Check sheet for the drawn part. Datum: minimum x, y, z corner. Units: mm. A direction names the side the tool comes from. Round coordinates to 2 decimals unless told otherwise and drop trailing zeros. Order: outer loops, then holes, each group sorted by start corner. A loop starts at its lowest first (then second) coordinate and runs counter-clockwise, first axis right, second up. Notation, with made-up numbers: (48, 45) -> (99, 45) arc R13 ccw to (99, 66) -> close; hole circle Ø6 at (62.25, -8.5). An arc over 180 degrees is marked (long way). Answer as a JSON object with one key per item and string values. Group by question number.
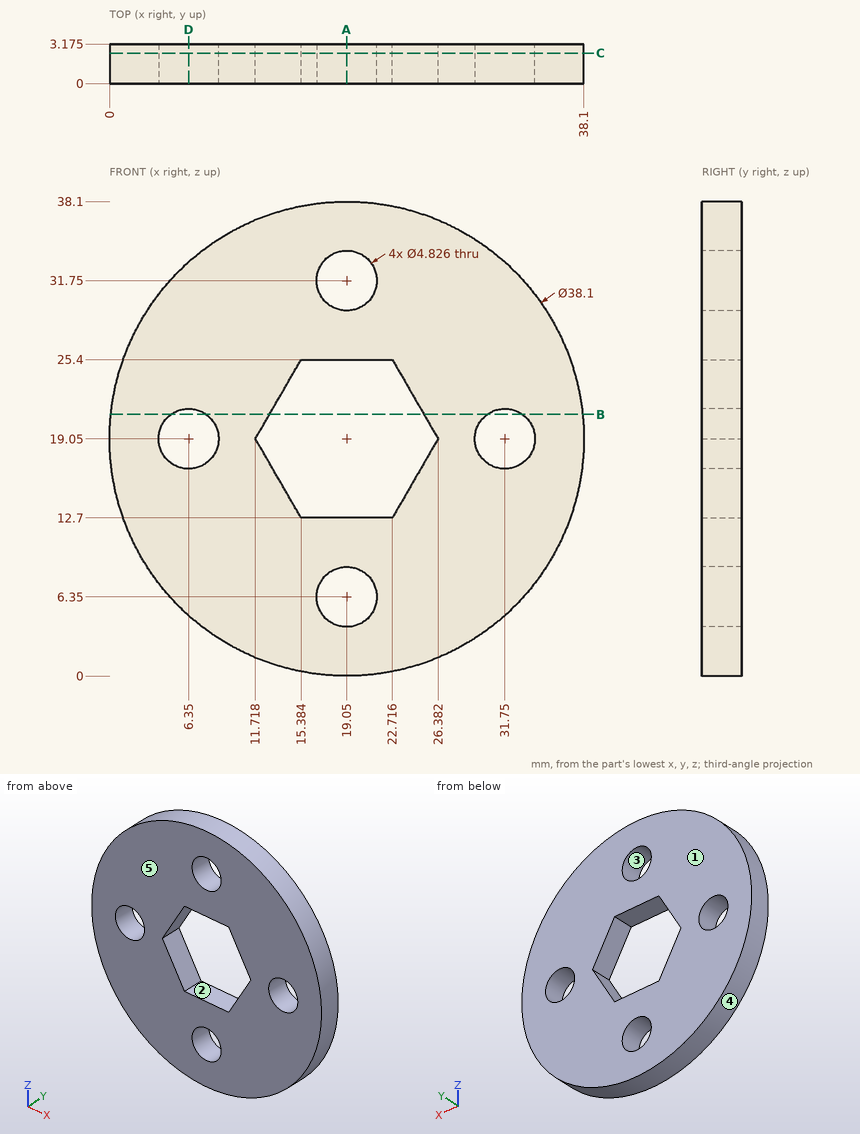
Item 1: Mould release check, pull along X, two halves, no side actions. Record for the marked faces 3, 4 and 5: pulls with the +X half, pulls with the -X half, needs draft (parallel to the pull), parting line crosses it, or undercut.
Item 2: Sectioned sample at D-D, the plane x = 6.35. Enter the section's corners in (y, z) (1 decimal).
Item 3: Depth check by flat-ended pin: pin 1 Ø1 at (x, y) = (19, 1) entering from +Z. Enter the tip coordinate at first touch or a pass-through.
Item 4: Sectioned sample at C-C, the plane y = 2.45. Enter the section's corners in (x, z), then the cut area to 3 significant figures.
Item 5: Sectioned sample at A-A, the plane x = 19.05. Enter the section's corners in (y, z) (1 decimal), then the cut area to 3 significant figures.
Item 6: Set-up check for the marked faces 1 and 2: record each of +Z, -Z, +X, -X, +Y, -Y from which the full face is reachable in a straight line by a thin tool's end or side.
Item 7: Sectioned sample at B-B, the plane z = 21. Enter the section's corners in (x, y) (1 decimal).
Item 8: Thickness scan on L1, parallel to X at y = 2.2, z = 19.05; L2, parallel to Z at x = 21, y = 2.5; L3, parallel to Z at x = 7.5, y = 2.5. Record the ranges inside material, lowest first.
Result:
{
 "1": {"face 3": "undercut", "face 4": "parting line crosses it", "face 5": "needs draft"},
 "2": {"outline": "(0, 4.9) -> (3.2, 4.9) -> (3.2, 16.6) -> (0, 16.6) -> close; (0, 21.5) -> (3.2, 21.5) -> (3.2, 33.2) -> (0, 33.2) -> close"},
 "3": {"pin 1": "stops at z = 38.1"},
 "4": {"outline": "circle Ø38.1 at (19.05, 19.05); hole circle Ø4.83 at (6.35, 19.05); hole (11.72, 19.05) -> (15.38, 12.7) -> (22.72, 12.7) -> (26.38, 19.05) -> (22.72, 25.4) -> (15.38, 25.4) -> close; hole circle Ø4.83 at (19.05, 6.35); hole circle Ø4.83 at (19.05, 31.75); hole circle Ø4.83 at (31.75, 19.05)", "area": "927 mm2"},
 "5": {"outline": "(0, 0) -> (3.2, 0) -> (3.2, 3.9) -> (0, 3.9) -> close; (0, 8.8) -> (3.2, 8.8) -> (3.2, 12.7) -> (0, 12.7) -> close; (0, 25.4) -> (3.2, 25.4) -> (3.2, 29.3) -> (0, 29.3) -> close; (0, 34.2) -> (3.2, 34.2) -> (3.2, 38.1) -> (0, 38.1) -> close", "area": "50.0 mm2"},
 "6": {"face 1": "+Z, -Z, +X, -X, +Y", "face 2": "+Y, -Y"},
 "7": {"outline": "(0.1, 0) -> (4.9, 0) -> (4.9, 3.2) -> (0.1, 3.2) -> close; (7.8, 0) -> (12.8, 0) -> (12.8, 3.2) -> (7.8, 3.2) -> close; (25.3, 0) -> (30.3, 0) -> (30.3, 3.2) -> (25.3, 3.2) -> close; (33.2, 0) -> (38, 0) -> (38, 3.2) -> (33.2, 3.2) -> close"},
 "8": {"L1": "x = 0 to 3.94, 8.76 to 11.72, 26.38 to 29.34, 34.16 to 38.1", "L2": "z = 0.1 to 4.93, 7.77 to 12.7, 25.4 to 30.33, 33.17 to 38", "L3": "z = 3.9 to 16.93, 21.17 to 34.2"}
}
